from build123d import *

# Parameters (mm, degrees)
CYLINDER006_R     = 2
CYLINDER006_DEPTH = 20
CYLINDER007_R     = 2
CYLINDER007_DEPTH = 20
CYLINDER005_R     = 2
CYLINDER005_DEPTH = 20
EXTRUDE003_DEPTH  = 16
EXTRUDE002_DEPTH  = 16
EXTRUDE001_DEPTH  = 16
CYLINDER004_R     = 2
CYLINDER004_DEPTH = 25
CYLINDER003_R     = 2
CYLINDER003_DEPTH = 25
CYLINDER002_R     = 2
CYLINDER002_DEPTH = 25
CYLINDER001_R     = 20
CYLINDER001_DEPTH = 5
CYLINDER_R        = 45
CYLINDER_DEPTH    = 20
EXTRUDE_DEPTH     = 25


with BuildPart() as cylinder006:
    # Cylinder006 → Cylinder006 (new body)
    with BuildSketch(Plane(origin=(-31, 18, 0), x_dir=(1, 0, 0), z_dir=(0, 0, 1))):
        Circle(CYLINDER006_R)
    extrude(amount=CYLINDER006_DEPTH)


with BuildPart() as cylinder007:
    # Cylinder007 → Cylinder007 (new body)
    with BuildSketch(Plane(origin=(0, -36, 0), x_dir=(1, 0, 0), z_dir=(0, 0, 1))):
        Circle(CYLINDER007_R)
    extrude(amount=CYLINDER007_DEPTH)


with BuildPart() as cylinder005:
    # Cylinder005 → Cylinder005 (new body)
    with BuildSketch(Plane(origin=(31, 18, 0), x_dir=(1, 0, 0), z_dir=(0, 0, 1))):
        Circle(CYLINDER005_R)
    extrude(amount=CYLINDER005_DEPTH)


with BuildPart() as extrude003:
    # RegularPolygon002 → Extrude003 (new body)
    with BuildSketch(Plane(origin=(46, -18, 0), x_dir=(0, 1, 0), z_dir=(0, 0, 1))):
        Polygon((0, -4.4), (3.810512, -2.2), (3.810512, 2.2), (0, 4.4), (-3.810512, 2.2), (-3.810512, -2.2), align=None)
    extrude(amount=EXTRUDE003_DEPTH)


with BuildPart() as extrude002:
    # RegularPolygon001 → Extrude002 (new body)
    with BuildSketch(Plane(origin=(-9, 48, 0), x_dir=(0, 1, 0), z_dir=(0, 0, 1))):
        Polygon((0, -4.4), (3.810512, -2.2), (3.810512, 2.2), (0, 4.4), (-3.810512, 2.2), (-3.810512, -2.2), align=None)
    extrude(amount=EXTRUDE002_DEPTH)


with BuildPart() as extrude001:
    # RegularPolygon → Extrude001 (new body)
    with BuildSketch(Plane(origin=(-38, -32, 0), x_dir=(0, 1, 0), z_dir=(0, 0, 1))):
        Polygon((0, -4.4), (3.810512, -2.2), (3.810512, 2.2), (0, 4.4), (-3.810512, 2.2), (-3.810512, -2.2), align=None)
    extrude(amount=EXTRUDE001_DEPTH)


with BuildPart() as cylinder004:
    # Cylinder004 → Cylinder004 (new body)
    with BuildSketch(Plane(origin=(46, -18, 0), x_dir=(1, 0, 0), z_dir=(0, 0, 1))):
        Circle(CYLINDER004_R)
    extrude(amount=CYLINDER004_DEPTH)


with BuildPart() as cylinder003:
    # Cylinder003 → Cylinder003 (new body)
    with BuildSketch(Plane(origin=(-9, 48, 0), x_dir=(1, 0, 0), z_dir=(0, 0, 1))):
        Circle(CYLINDER003_R)
    extrude(amount=CYLINDER003_DEPTH)


with BuildPart() as cylinder002:
    # Cylinder002 → Cylinder002 (new body)
    with BuildSketch(Plane(origin=(-38, -32, 0), x_dir=(1, 0, 0), z_dir=(0, 0, 1))):
        Circle(CYLINDER002_R)
    extrude(amount=CYLINDER002_DEPTH)


with BuildPart() as cylinder001:
    # Cylinder001 → Cylinder001 (new body)
    with BuildSketch(Plane.XY):
        Circle(CYLINDER001_R)
    extrude(amount=CYLINDER001_DEPTH)


with BuildPart() as cylinder:
    # Cylinder → Cylinder (new body)
    with BuildSketch(Plane.XY.offset(5)):
        Circle(CYLINDER_R)
    extrude(amount=CYLINDER_DEPTH)


with BuildPart() as cut010:
    # Sketch → Extrude (new body)
    with BuildSketch(Plane.XY):
        with BuildLine():
            ThreePointArc((-58.518876, 0), (-47.172244, -27.235666), (-29.233044, -50.660282))
            ThreePointArc((-29.233044, -50.660282), (0.013292, -54.368862), (29.263356, -50.689798))
            ThreePointArc((29.263356, -50.689798), (47.126286, -27.222202), (58.473712, 0))
            ThreePointArc((58.473712, 0), (47.267042, 27.297009), (29.223904, 50.645699))
            ThreePointArc((29.223904, 50.645699), (-0.099691, 54.190035), (-29.41792, 50.601573))
            ThreePointArc((-29.41792, 50.601573), (-47.081429, 27.09109), (-58.518876, 0))
        make_face()
    extrude(amount=EXTRUDE_DEPTH)

    # Cut: cut Cylinder
    add(cylinder.part, mode=Mode.SUBTRACT)

    # Cut001: cut Cylinder001
    add(cylinder001.part, mode=Mode.SUBTRACT)

    # Cut002: cut Cylinder002
    add(cylinder002.part, mode=Mode.SUBTRACT)

    # Cut003: cut Cylinder003
    add(cylinder003.part, mode=Mode.SUBTRACT)

    # Cut004: cut Cylinder004
    add(cylinder004.part, mode=Mode.SUBTRACT)

    # Cut005: cut Extrude001
    add(extrude001.part, mode=Mode.SUBTRACT)

    # Cut006: cut Extrude002
    add(extrude002.part, mode=Mode.SUBTRACT)

    # Cut007: cut Extrude003
    add(extrude003.part, mode=Mode.SUBTRACT)

    # Cut008: cut Cylinder005
    add(cylinder005.part, mode=Mode.SUBTRACT)

    # Cut009: cut Cylinder007
    add(cylinder007.part, mode=Mode.SUBTRACT)

    # Cut010: cut Cylinder006
    add(cylinder006.part, mode=Mode.SUBTRACT)


solid = cut010.part
Geometry check sheet. Reference: the model listing, model coordinates, mm. A direction names the side the tool comes from. Give positions to 0.01 mm unless a question says otherwise; leave off trailing zeros. Order: outer loops, then holes, each group sorted by start corner. A loop starts at its lowest first (then second) coordinate and runs counter-clockwise, first axis right, second up.
1) Cross-section at A-A (z = 3.5). Record the boundary of the cut face in (x, y), then the cut area to 3 significant figures.
Results are:
outline: (-58.52, 0) arc R114.32 ccw to (-29.23, -50.66) arc R117.64 ccw to (29.26, -50.69) arc R115.67 ccw to (58.47, 0) arc R110.29 ccw to (29.22, 50.65) arc R122.31 ccw to (-29.42, 50.6) arc R120.4 ccw to start; hole (-42.4, -32) - (-40.2, -35.81) - (-35.8, -35.81) - (-33.6, -32) - (-35.8, -28.19) - (-40.2, -28.19) - close; hole circle Ø4 at (-31, 18); hole circle Ø40 at (0, 0); hole (-13.4, 48) - (-11.2, 44.19) - (-6.8, 44.19) - (-4.6, 48) - (-6.8, 51.81) - (-11.2, 51.81) - close; hole circle Ø4 at (0, -36); hole circle Ø4 at (31, 18); hole (41.6, -18) - (43.8, -21.81) - (48.2, -21.81) - (50.4, -18) - (48.2, -14.19) - (43.8, -14.19) - close
area: 8,320 mm2
2) Gauge pin test, flat ends, axial feed: pin 1 (4.5 mm diameter, centred on x = 0, y = -36, fed in from -Z); pin 2 (8 mm diameter, centred on x = -35.5, z = 4, fed in from -Y); pin 3 (10 mm diameter, centred on x = 12, z = 14, fed in from -Y); pin 4 (2 mm diameter, centred on x = 45.5, z = 4.5, fed in from +Y). Record the tip position at first contact, or that the pin passes through.
Results are:
pin 1: stops at z = 0
pin 2: stops at y = -48.32
pin 3: stops at y = -54.16
pin 4: stops at y = 31.83
3) Cross-section at C-C (z = 18.5). Record the boundary of the cut face in (x, y), then the cut area to 3 significant figures.
Results are:
outline: (-58.52, 0) arc R114.32 ccw to (-29.23, -50.66) arc R117.64 ccw to (29.26, -50.69) arc R115.67 ccw to (58.47, 0) arc R110.29 ccw to (29.22, 50.65) arc R122.31 ccw to (-29.42, 50.6) arc R120.4 ccw to start; hole circle Ø90 at (0, 0); hole circle Ø4 at (-38, -32); hole circle Ø4 at (-9, 48); hole circle Ø4 at (46, -18)
area: 3,370 mm2
4) Draft check along X on faces 4 (the cylindrical face through (47.474, 26.938, 12.325)), 5 (the flat face through (-38, -28.189, 8)), 6 (the cylindrical face through (-0.401, -54.368, 12.325)). Enter one of: released by +X, released by -X, zero draft, split by the parting line, or undercut.
Results are:
face 4: released by +X
face 5: undercut
face 6: split by the parting line
5) Tool access check on faces 1 (the cylindrical face through (46.92, -27.58, 12.32)), 2 (the flat face through (-34.715, -33.932, 7.888)), 3 (the flat face through (9, -19, 5)). Record the directions out of +Z, -Z, +X, -X, +Y, -Y that give a thin tool (end or side, any length) a straight path to the whole face; none if there is none.
Results are:
face 1: +Z, -Z, +X, -Y
face 2: -Z
face 3: +Z
6) Material ranges on probe 1 along Y at (x, z) = (0, 3.5); probe 2 along X at (y, z) = (0, 20.5); probe 3 along Z at (x, y) = (-7.5, -20), recorded low to high.
Results are:
probe 1: y = -54.37 to -38, -34 to -20, 20 to 54.19
probe 2: x = -58.52 to -45, 45 to 58.47
probe 3: z = 0 to 5
7) Cross-section at D-D (y = 22). Record the boundary of the cut face in (x, z).
Results are:
outline: (-49.85, 0) - (50.14, 0) - (50.14, 25) - (39.26, 25) - (39.26, 5) - (-39.26, 5) - (-39.26, 25) - (-49.85, 25) - close
8) Cross-section at B-B (x = -38). Record the boundary of the cut face in (y, z).
Results are:
outline: (-40.77, 0) - (-35.81, 0) - (-35.81, 16) - (-34, 16) - (-34, 25) - (-40.77, 25) - close; (-30, 16) - (-28.19, 16) - (-28.19, 0) - (40.66, 0) - (40.66, 25) - (24.1, 25) - (24.1, 5) - (-24.1, 5) - (-24.1, 25) - (-30, 25) - close
